Read the model definition and answer for the solid it produces. Units are mm, in the model's axes. A direction names the side the tool comes from. Coordinates: 2 decimals unless noted, no trailing zeros. Write each loop counter-clockwise with the first axis right and the second up, starting at its lowest first coordinate (ties: lowest second). Pieces come first, ordered by that corner, then holes.
(1) Given pin 1 (8 mm diameter, centred on x = 46.5, y = 11.5, fed in from -Z); pin 2 (5 mm diameter, centred on x = 47, z = 44.5, fed in from -Y); pin 3 (16.5 mm diameter, centred on x = -78.5, y = 2.5, fed in from +Z); pin 4 (6 mm diameter, centred on x = -59, y = -24.5, fed in from +Z), each flat-ended and moving along its own axis, determine where each tip first touches the part or whether it passes through.
(2) Section D-D on y = -24 is taken. Write down the section's boundary in (x, z), then the cut area to 3 significant figures.
(3) Section B-B on z = 23 is taken. Write down the section's boundary in (x, y), then the cut area to 3 significant figures.
(4) Find the intervals of material crossed by probe 1 along X at (y, z) = (-1, 18); probe 2 along Z at (x, y) = (83.5, -12); probe 3 along Y at (x, z) = (80, 15), in increasing order.
(5) Section A-A on x = 0 is taken. Write down the section's boundary in (y, z), then the cut area to 3 significant figures.
(6) Section C-C on y = 0 is taken. State how many separate pieces and enclosed holes the cut face has, then the cut area to 3 significant figures.
(7) The mould has two halves that part along X. Classify faces 1 (the flat face through (-84.5, 9.9, 25)), 2 (the flat face through (50, 0, 11.5)), 3 (the flat face through (-53.138, -29.548, 5.67)): +X half, -X half, draft (parallel to the pull), parting line (faces both ways), or undercut.
(8) Which of the six approach directions +Z, -Z, +X, -X, +Y, -Y give full straight-line access (tool end or side, diameter ignored) to faces 4 (the flat face through (84.5, -9.9, 25)), 5 (the flat face through (52.19, -29.95, 5.67)), 6 (the cylindrical face through (-96.44, 2.74, 15.1))?
from build123d import *

# Parameters (mm, degrees)
BOSS_EXTRUDE1_DEPTH   = 11.5
BOSS_EXTRUDE1_2_DEPTH = 11.5
CUT_EXTRUDE1_DEPTH    = 2.5
SKETCH1_4_R           = 16.666666667
SKETCH1_4_R_2         = 10.666666667
BOSS_EXTRUDE2_DEPTH   = 25
SKETCH1_5_R           = 48
SKETCH1_5_R_2         = 42
BOSS_EXTRUDE3_DEPTH   = 63


with BuildPart() as part:
    # Sketch1 → Boss-Extrude1 (new body)
    with BuildSketch(Plane.XY):
        with BuildLine():
            Line((-86.527777778, -15.335119662), (-18.8, -44.165144628))
            ThreePointArc((-18.8, -44.165144628), (-48, 0), (-18.8, 44.165144628))
            Line((-18.8, 44.165144628), (-86.527777778, 15.335119662))
            ThreePointArc((-86.527777778, 15.335119662), (-70.808115496, 13.90277084), (-63.333333333, 0))
            ThreePointArc((-63.333333333, 0), (-70.808115496, -13.90277084), (-86.527777778, -15.335119662))
        make_face()
    extrude(amount=BOSS_EXTRUDE1_DEPTH)

    # Sketch2 → Cut-Extrude1 (cut)
    with BuildSketch(Plane.XY.offset(11.5)):
        with BuildLine():
            Line((-46.329311604, 29.72952886), (-68.749829189, 20.185673992))
            ThreePointArc((-68.749829189, 20.185673992), (-70.258507425, 18.131633045), (-69.181739923, 15.821705345))
            ThreePointArc((-69.181739923, 15.821705345), (-60.833333333, 0), (-69.181739923, -15.821705345))
            ThreePointArc((-69.181739923, -15.821705345), (-70.258507425, -18.131633045), (-68.749829189, -20.185673992))
            Line((-68.749829189, -20.185673992), (-46.329311604, -29.72952886))
            ThreePointArc((-46.329311604, -29.72952886), (-43.461816215, -29.067618209), (-43.210987158, -26.135427849))
            ThreePointArc((-43.210987158, -26.135427849), (-50.5, 0), (-43.210987158, 26.135427849))
            ThreePointArc((-43.210987158, 26.135427849), (-43.461816215, 29.067618209), (-46.329311604, 29.72952886))
        make_face()
    cut_extrude1 = extrude(amount=-CUT_EXTRUDE1_DEPTH, mode=Mode.SUBTRACT)



with BuildPart() as body_2:
    # Sketch1 → Boss-Extrude1 2 (new body)
    with BuildSketch(Plane.XY):
        with BuildLine():
            ThreePointArc((48, 0), (40.03998002, -26.472627372), (18.8, -44.165144628))
            Line((18.8, -44.165144628), (86.527777778, -15.335119662))
            ThreePointArc((86.527777778, -15.335119662), (63.333333333, 0), (86.527777778, 15.335119662))
            Line((86.527777778, 15.335119662), (18.8, 44.165144628))
            ThreePointArc((18.8, 44.165144628), (40.03998002, 26.472627372), (48, 0))
        make_face()
    extrude(amount=BOSS_EXTRUDE1_2_DEPTH)

    # Mirror1: Cut-Extrude1 across plane
    add(cut_extrude1.mirror(Plane(origin=(0, 0, 0), x_dir=(0, 0, 1), z_dir=(1, 0, 0))), mode=Mode.SUBTRACT)


with BuildPart() as part_1:
    add(part.part)

    add(body_2.part)  # Boss-Extrude2 merges body 2
    # Sketch1_4 → Boss-Extrude2 (add)
    # profile 1 of 2: a face of its own
    with BuildSketch(Plane.XY):
        with Locations(Location((-80, 0, 0), (0, 0, 113.058244088))):
            Circle(SKETCH1_4_R)
        with Locations((-80, 0)):
            Circle(SKETCH1_4_R_2, mode=Mode.SUBTRACT)
    # profile 2 of 2: a face of its own
    with BuildSketch(Plane.XY):
        with Locations(Location((80, 0, 0), (0, 0, 293.058244088))):
            Circle(SKETCH1_4_R)
        with Locations((80, 0)):
            Circle(SKETCH1_4_R_2, mode=Mode.SUBTRACT)
    extrude(amount=BOSS_EXTRUDE2_DEPTH)

    # Sketch1_5 → Boss-Extrude3 (add)
    with BuildSketch(Plane.XY):
        with Locations(Location((0, 0, 0), (0, 0, 113.058244088))):
            Circle(SKETCH1_5_R)
        Circle(SKETCH1_5_R_2, mode=Mode.SUBTRACT)
    extrude(amount=BOSS_EXTRUDE3_DEPTH)


solid = part_1.part
Response:
1. pin 1: stops at z = 0
1. pin 2: stops at y = -17.99
1. pin 3: stops at z = 25
1. pin 4: stops at z = 11.5
2. outline: (-66.17, 0) - (-34.47, 0) - (-34.47, 63) - (-41.57, 63) - (-41.57, 11.5) - (-44.43, 11.5) - (-44.43, 9) - (-59.79, 9) - (-59.79, 11.5) - (-66.17, 11.5) - close; (34.47, 0) - (66.17, 0) - (66.17, 11.5) - (59.79, 11.5) - (59.79, 9) - (44.43, 9) - (44.43, 11.5) - (41.57, 11.5) - (41.57, 63) - (34.47, 63) - close
2. area: 1,380 mm2
3. outline: circle Ø33.33 at (-80, 0); circle Ø96 at (0, 0); circle Ø33.33 at (80, 0); hole circle Ø21.33 at (-80, 0); hole circle Ø84 at (0, 0); hole circle Ø21.33 at (80, 0)
3. area: 2,730 mm2
4. probe 1: x = -96.64 to -90.62, -69.38 to -63.36, -47.99 to -41.99, 41.99 to 47.99, 63.36 to 69.38, 90.62 to 96.64
4. probe 2: z = 0 to 25
4. probe 3: y = -16.67 to -10.67, 10.67 to 16.67
5. outline: (-48, 0) - (-42, 0) - (-42, 63) - (-48, 63) - close; (42, 0) - (48, 0) - (48, 63) - (42, 63) - close
5. area: 756 mm2
6. separate pieces: 4
6. enclosed holes: 0
6. area: 1,660 mm2
7. face 1: draft
7. face 2: undercut
7. face 3: -X half
8. face 4: +Z, +X, +Y, -Y
8. face 5: +Z, -Z, +X, -Y
8. face 6: +Z
